Autodesk Inventor part; units mm, degrees
ref_plane "YZ Plane" through (0, 0, 0) normal (1, 0, 0) x (0, 1, 0)
ref_plane "XZ Plane" through (0, 0, 0) normal (0, 1, 0) x (-1, 0, 0)
ref_plane "XY Plane" through (0, 0, 0) normal (0, 0, 1) x (1, 0, 0)
sketch "Sketch1" plane through (0, 0, 0) normal (0, 1, 0) x (-1, 0, 0)
  line L0 (0, 0) -> (93.0623, 0)
  line L1 (93.0623, 0) -> (93.0623, -128.95)
  line L2 (93.0623, -128.95) -> (0, -128.95)
  line L3 (0, -128.95) -> (0, 0)
  dimension "d0" = 93.0623
  dimension "d1" = 128.95
extrude "Extrusion1" add sketch "Sketch1" along normal blind 3.2
sketch "Sketch2" plane through (0, 3.2, 0) normal (0, 1, 0) x (1, 0, 0)
  line L0 (-73.2061, 115.27) -> (-19.8561, 115.27)
  line L1 (-19.8561, 115.27) -> (-19.8561, 13.68)
  line L2 (-19.8561, 13.68) -> (-73.2061, 13.68)
  line L3 (-73.2061, 13.68) -> (-73.2061, 115.27)
  circle A0 centre (-70.6561, 28.92) radius 1.5875
  circle A1 centre (-22.3961, 27.65) radius 1.5875
  circle A2 centre (-22.3961, 110.2) radius 1.5875
  circle A3 centre (-70.6561, 103.85) radius 1.5875
  circle A4 centre (-27.4761, 79.72) radius 1.5875
  line L4 (-93.0623, 0) -> (0, 0)
  line L5 (-93.0623, 128.95) -> (-93.0623, 0)
  line L6 (0, 128.95) -> (-93.0623, 128.95)
  line L7 (-76.4061, 118.47) -> (-16.6561, 118.47)
  line L8 (-16.6561, 118.47) -> (-16.6561, 10.48)
  line L9 (-16.6561, 10.48) -> (-76.4061, 10.48)
  line L10 (-76.4061, 10.48) -> (-76.4061, 118.47)
  dimension "d4" = 101.59
  dimension "d5" = 53.35
  dimension "d6" = 15.24
  dimension "d7" = 3.175
  dimension "d8" = 50.8
  dimension "d9" = 13.97
  dimension "d10" = 2.54
  dimension "d11" = 90.17
  dimension "d12" = 96.52
  dimension "d13" = 50.8
  dimension "d14" = 2.54
  dimension "d15" = 66.04
  dimension "d16" = 7.62
  dimension "d20" = 93.0623
  dimension "d21" = 19.8561
  dimension "d22" = 128.95
  dimension "d23" = 13.68
  dimension "d26" = 3.2
  dimension "d27" = 3.2
  dimension "d28" = 3.2
  dimension "d29" = 3.2
extrude "Extrusion2" cut sketch "Sketch2" against normal up to surface (3.2 mm away) contours A0 | A1 | A2 | A3 | A4
sketch "Sketch3" plane through (0, 3.2, 0) normal (0, 1, 0) x (1, 0, 0)
  line L0 (-76.4061, 10.48) -> (-76.4061, 118.47)
  line L1 (-73.2061, 13.68) -> (-73.2061, 115.27)
  line L2 (-19.8561, 13.68) -> (-73.2061, 13.68)
  line L3 (-16.6561, 10.48) -> (-76.4061, 10.48)
  line L4 (-16.6561, 118.47) -> (-16.6561, 10.48)
  line L5 (-73.2061, 115.27) -> (-19.8561, 115.27)
  line L6 (-76.4061, 118.47) -> (-16.6561, 118.47)
  line L7 (-19.8561, 115.27) -> (-19.8561, 13.68)
  point P0 (0, 0)
extrude "Extrusion3" cut sketch "Sketch3" against normal blind 1
sketch "Sketch4" plane through (0, 3.2, 0) normal (0, 1, 0) x (1, 0, 0)
  line L0 (-93.0623, 0) -> (0, 0)
  line L1 (-89.8623, 0) -> (-3.2, 0)
  line L2 (-3.2, 0) -> (-3.2, -5)
  line L3 (-3.2, -5) -> (-89.8623, -5)
  line L4 (-89.8623, -5) -> (-89.8623, 0)
  line L5 (0, 128.95) -> (-93.0623, 128.95)
  line L6 (-89.8623, 128.95) -> (-3.2, 128.95)
  line L7 (-3.2, 128.95) -> (-3.2, 133.95)
  line L8 (-3.2, 133.95) -> (-89.8623, 133.95)
  line L9 (-89.8623, 133.95) -> (-89.8623, 128.95)
  line L10 (-93.0623, 128.95) -> (-93.0623, 0)
  line L11 (0, 0) -> (0, 128.95)
  dimension "d32" = 3.2
  dimension "d33" = 3.2
  dimension "d34" = 5
  dimension "d35" = 5
extrude "Extrusion4" add sketch "Sketch4" against normal up to surface (3.2 mm away) contours L0 L2 L3 L4 | L9 L8 L7 L5
equation "\"d1\" = largo_abdomen_robot - acople_hombro_grosor_trasero"
equation "\"d13\" = d8"
equation "\"d14\" = d10"
equation "\"d21\" = -0.5 * d5 + 0.5 * d20"
equation "\"d23\" = -0.5 * d4 + 0.5 * d22"
equation "\"d27\" = d26"
equation "\"d28\" = d26"
equation "\"d29\" = d28"
equation "\"d33\" = d32"
equation "\"d35\" = d34"
properties part number "Cuerpo - Base Arduino"
Geometry check sheet. Reference: the model listing, model coordinates, mm. A direction names the side the tool comes from. Round coordinates to 2 decimals unless told otherwise and drop trailing zeros. Order: outer loops, then holes, each group sorted by start corner. A loop starts at its lowest first (then second) coordinate and runs counter-clockwise, first axis right, second up. Notation, with made-up numbers: M -31.75,19 L 2.25,19 A12 ccw 2.25,24 Z; hole C -27,-34 d1. An arc over 180 degrees is marked long. Answer in a Markdown table with one row per item. Add a question column.
Item 1: Draft check along X on faces 1 (the face through (-21.543, 1.622, -28.989)), 2 (the face through (-46, 3.2, -64)), 3 (the face through (-22.74, 1.62, -108.65)), 4 (the face through (0, 2, -65)). Enter one of: released by +X, released by -X, zero draft, split by the parting line, or undercut.
Item 2: Set-up check for faces 5 (the face through (-91, 2, 0)), 6 (the face through (-2, 2, -128.95)), 7 (the face through (-75, 2.2, -61)), 8 (the face through (-3.2, 2, 2)), 9 (the face through (-91, 2, -128.95)): record each of +Z, -Z, +X, -X, +Y, -Y from which the full face is reachable in a straight line by a thin tool's end or side.
Item 3: Material ranges on L1, parallel to X at y = 2.7, z = -22; L2, parallel to X at y = 1.3, z = -28.92; L3, parallel to Y at x = -17, z = -56.5, recorded low to high. Write a range as [from, to].
Item 4: Depth check by flat-ended pin: pin 1 Ø1.5 at (x, z) = (-29.5, -20) entering from -Y; pin 2 Ø2.5 at (x, z) = (-22.4, -110.2) entering from -Y; pin 3 Ø1 at (y, z) = (2, -132) entering from -X; pin 4 Ø1 at (x, y) = (-2, 1) entering from +Z. Enter the tip coordinate at first touch or a pass-through.
Item 5: Sectioned sample at B-B, the plane z = -48. Enter the section's corners in (x, y).
Item 6: Sectioned sample at A-A, the plane z = -79.72. Enter the section's corners in (x, y), plus the area to 3 significant figures.
Filled in:
| question | item | result |
|---|---|---|
| 1 | face 1 | undercut |
| 1 | face 2 | zero draft |
| 1 | face 3 | undercut |
| 1 | face 4 | released by +X |
| 2 | face 5 | +Z, -X, +Y, -Y |
| 2 | face 6 | -Z, +X, +Y, -Y |
| 2 | face 7 | +Y |
| 2 | face 8 | +Z, +X, +Y, -Y |
| 2 | face 9 | -Z, -X, +Y, -Y |
| 3 | L1 | x = [-93.06, -76.41], [-73.21, -19.86], [-16.66, 0] |
| 3 | L2 | x = [-93.06, -72.24], [-69.07, -23.35], [-21.44, 0] |
| 3 | L3 | y = [0, 2.2] |
| 4 | pin 1 | stops at y = 0 |
| 4 | pin 2 | passes through |
| 4 | pin 3 | stops at x = -89.86 |
| 4 | pin 4 | stops at z = 0 |
| 5 | outline | M -93.06,0 L 0,0 L 0,3.2 L -16.66,3.2 L -16.66,2.2 L -19.86,2.2 L -19.86,3.2 L -73.21,3.2 L -73.21,2.2 L -76.41,2.2 L -76.41,3.2 L -93.06,3.2 Z |
| 6 | outline | M -93.06,0 L -29.06,0 L -29.06,3.2 L -73.21,3.2 L -73.21,2.2 L -76.41,2.2 L -76.41,3.2 L -93.06,3.2 Z; M -25.89,0 L 0,0 L 0,3.2 L -16.66,3.2 L -16.66,2.2 L -19.86,2.2 L -19.86,3.2 L -25.89,3.2 Z |
| 6 | area | 281 mm² |
